The drawing under review shows one solid part. Ordinate dimensions are in mm from its lowest x, y, z. A direction names the side the tool comes from. Give positions to 0.01 mm unless a question says otherwise; leave off trailing zeros. Write each loop counter-clockwise with the first axis right and the second up, starting at its lowest first coordinate (ties: lowest second). Pieces come first, ordered by that corner, then holes.
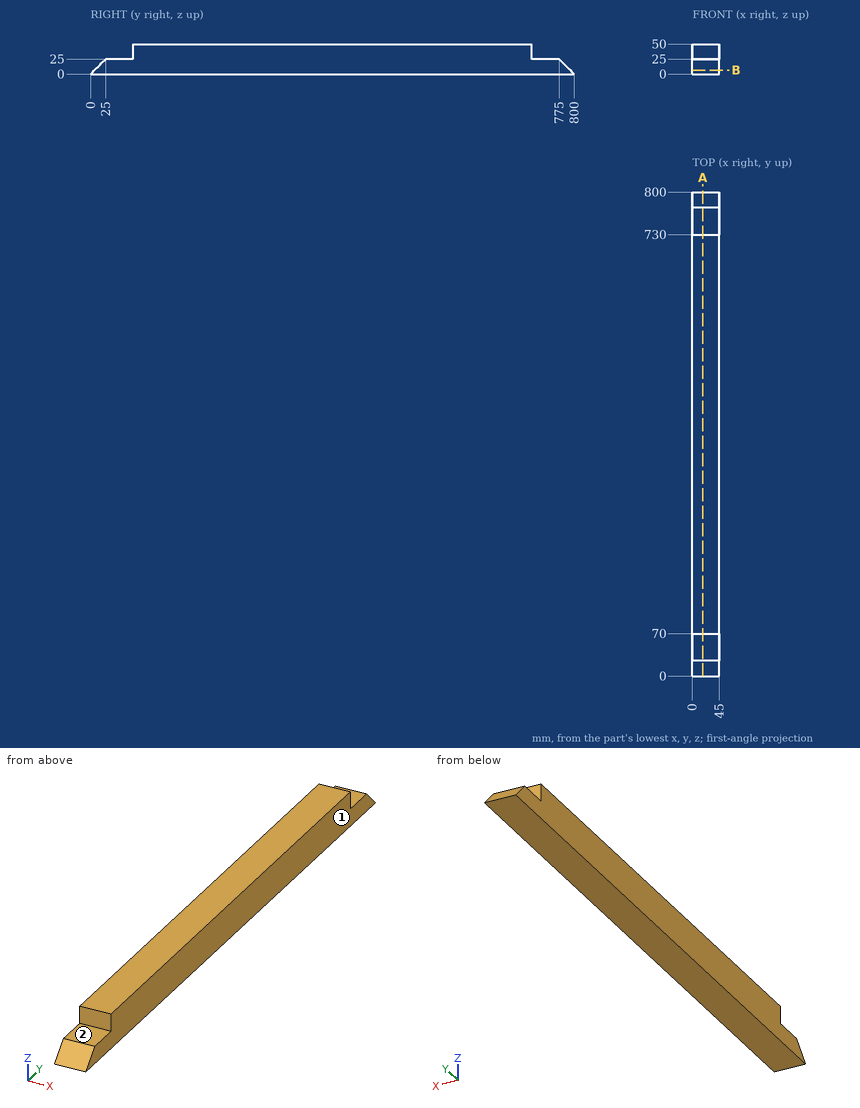
1) Consider section A-A, the plane x = 17.5. Give the boundary of the cut face in (y, z).
2) Tool access review of the marked faces 1 and 2: name each direction out of +Z, -Z, +X, -X, +Y, -Y from which nothing blocks a thin tool from reaching the whole face with its end or side.
3) Consider section B-B, the plane z = 7. Give the boundary of the cut face in (x, y), then the cut area to 3 significant figures.
4) To check wall thickness, follow probe 1 along Y at (x, z) = (40, 27); probe 2 along Z at (x, y) = (6, 56); probe 3 along Y at (x, z) = (16, 22.5). State the ranges of each line that lie inside material, in increasing order.
5) Insertion check: pin 1 (12.5 mm diameter, centred on x = 17, z = 43, fed in from +Y); pin 2 (22.5 mm diameter, centred on x = 27, y = 49, fed in from +Z); pin 3 (12.5 mm diameter, centred on x = 24.5, z = 35.5, fed in from -Y). Each pin has a flat end and moves straight along its axis. Give the tip position at first contact, or say it passes through.
Answer block:
1. outline: (0, 0) - (800, 0) - (775, 25) - (730, 25) - (730, 50) - (70, 50) - (70, 25) - (25, 25) - close
2. face 1: +Z, -Z, +X, +Y, -Y
2. face 2: +Z, +X, -X, -Y
3. outline: (0, 7) - (45, 7) - (45, 793) - (0, 793) - close
3. area: 35,400 mm2
4. probe 1: y = 70 to 730
4. probe 2: z = 0 to 25
4. probe 3: y = 22.5 to 777.5
5. pin 1: stops at y = 730
5. pin 2: stops at z = 25
5. pin 3: stops at y = 70
